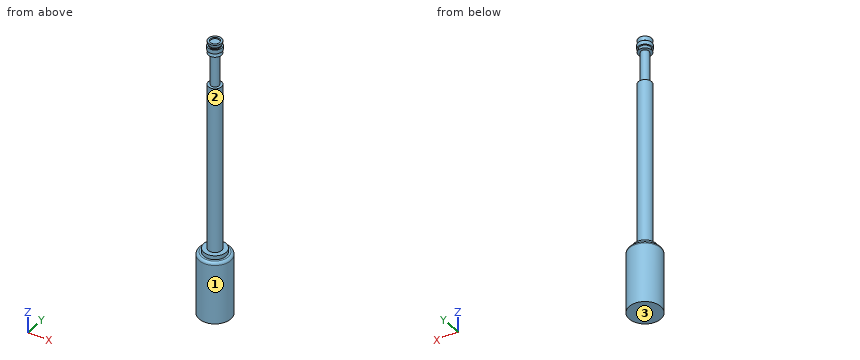
```python
from build123d import *

# Parameters (mm, degrees)
SKETCH2_R           = 0.5
BOSS_EXTRUDE1_DEPTH = 15.5
SKETCH2_3_R         = 1.2
BOSS_EXTRUDE2_DEPTH = 4.75
FILLET1_R           = 0.2
SKETCH3_R           = 0.85
BOSS_EXTRUDE3_DEPTH = 0.3
SKETCH5_W           = 0.452483434
SKETCH5_H           = 0.029273323
SKETCH6_W           = 1.07619714
SKETCH6_H           = 2.46


with BuildPart() as part:
    # Sketch2 → Boss-Extrude1 (new body)
    with BuildSketch(Plane.XY):
        Circle(SKETCH2_R)
    extrude(amount=BOSS_EXTRUDE1_DEPTH)

    # Sketch2<3> → Boss-Extrude2 (add)
    with BuildSketch(Plane.XY):
        Circle(SKETCH2_3_R)
    extrude(amount=-BOSS_EXTRUDE2_DEPTH)

    # Fillet1
    fillet1_edges = [part.edges().sort_by_distance(p)[0] for p in [
        (-1.2, 0, 0),
    ]]
    fillet(fillet1_edges, radius=FILLET1_R)

    # Sketch3 → Boss-Extrude3 (add)
    with BuildSketch(Plane.XY):
        Circle(SKETCH3_R)
    extrude(amount=BOSS_EXTRUDE3_DEPTH)

    # Sketch4 → Revolve1 (revolve)
    with BuildSketch(Plane(origin=(0, 0, 0), x_dir=(1, 0, 0), z_dir=(0, 1, 0))):
        with BuildLine():
            Line((0.5, -15.5), (0, -15.5))
            Line((0, -15.5), (0, -16.0775))
            ThreePointArc((0, -16.0775), (0.247487373, -16.180012627), (0.35, -16.4275))
            Line((0.35, -16.4275), (0.5, -16.4275))
            ThreePointArc((0.5, -16.4275), (0.479947408, -16.287319809), (0.421398056, -16.158383523))
            Line((0.421398056, -16.158383523), (0.421398056, -16.076439057))
            Line((0.421398056, -16.076439057), (0.523845222, -16.076439057))
            Line((0.523845222, -16.076439057), (0.523845222, -15.778410938))
            Line((0.523845222, -15.778410938), (0.421398056, -15.778410938))
            ThreePointArc((0.421398056, -15.778410938), (0.441425242, -15.633764027), (0.5, -15.5))
        make_face()
    revolve(axis=Axis((0, 0, 15.5), (0, 0, 1)))

    # Sketch5 → Revolve2 (revolve)
    with BuildSketch(Plane(origin=(0, 0, 0), x_dir=(1, 0, 0), z_dir=(0, 1, 0))):
        with Locations((-0.226241717, -16.325363339)):
            Rectangle(SKETCH5_W, SKETCH5_H)
    revolve(axis=Axis((0, 0, 15.5), (0, 0, 1)))

    # Sketch6 → Cut-Revolve1 (revolve, cut)
    with BuildSketch(Plane(origin=(0, 0, 0), x_dir=(1, 0, 0), z_dir=(0, 1, 0))):
        with Locations((-0.83809857, -14.27)):
            Rectangle(SKETCH6_W, SKETCH6_H)
    revolve(axis=Axis((0, 0, 15.5), (0, 0, 1)), mode=Mode.SUBTRACT)


solid = part.part
```
Can you work these out from the model? Positions are in its coordinate system, mm. Face numbers are marked on the shaded views. Round coordinates to 2 decimals unless told otherwise and drop trailing zeros. Loops run counter-clockwise (first coordinate to the right, second up) from the corner with the lowest first, then second, coordinate; pieces in that order, holes last. Notation, with made-up numbers: M 26.5,-2 L 81.5,-2 A21 ccw 81.5,11 Z; hole C -26.5,4.5 d2. An arc over 180 degrees is marked long. Answer as a JSON object with one key per item and string values. Group by question number.
Q1. Imagine slicing it at B-B, the plane z = 8.5. Please give me the cut outline in (x, y).
Q2. Imagine slicing it at A-A, the plane z = -2.5. Please give me the cut outline in (x, y), then the cut area to 3 significant figures.
Q3. Please list where these lines run through material, in increasing order: L1, parallel to Z at x = -0.2, y = -0.55; L2, parallel to X at y = -0.4, z = 5.5; L3, parallel to X at y = 0.05, z = 9.25.
Q4. We'd pull the mould along Z, two halves only. Please class the marked faces 1, 2 and 3: +Z half, -Z half, draft (parallel to the pull), parting line (faces both ways), or undercut.
Q5. Will this pin go through, and if not, where does the flat tip stop? pin 1 (0.5 mm diameter, centred on x = 0, y = 0, fed in from +Z).
Findings:
{
 "1": {"outline": "C 0,0 d1"},
 "2": {"outline": "C 0,0 d2.4", "area": "4.52 mm2"},
 "3": {"L1": "z = -4.75 to 0.3", "L2": "x = -0.3 to 0.3", "L3": "x = -0.5 to 0.5"},
 "4": {"face 1": "draft", "face 2": "undercut", "face 3": "-Z half"},
 "5": {"pin 1": "stops at z = 16.34"}
}
